Design review of the part shown in the three views and the two pictorial views. Dimensions are in mm from the part's minimum x, y and z. A direction names the side the tool comes from. Coordinates: 2 decimals unless noted, no trailing zeros. Loops run counter-clockwise (first coordinate to the right, second up) from the corner with the lowest first, then second, coordinate; pieces in that order, holes last.
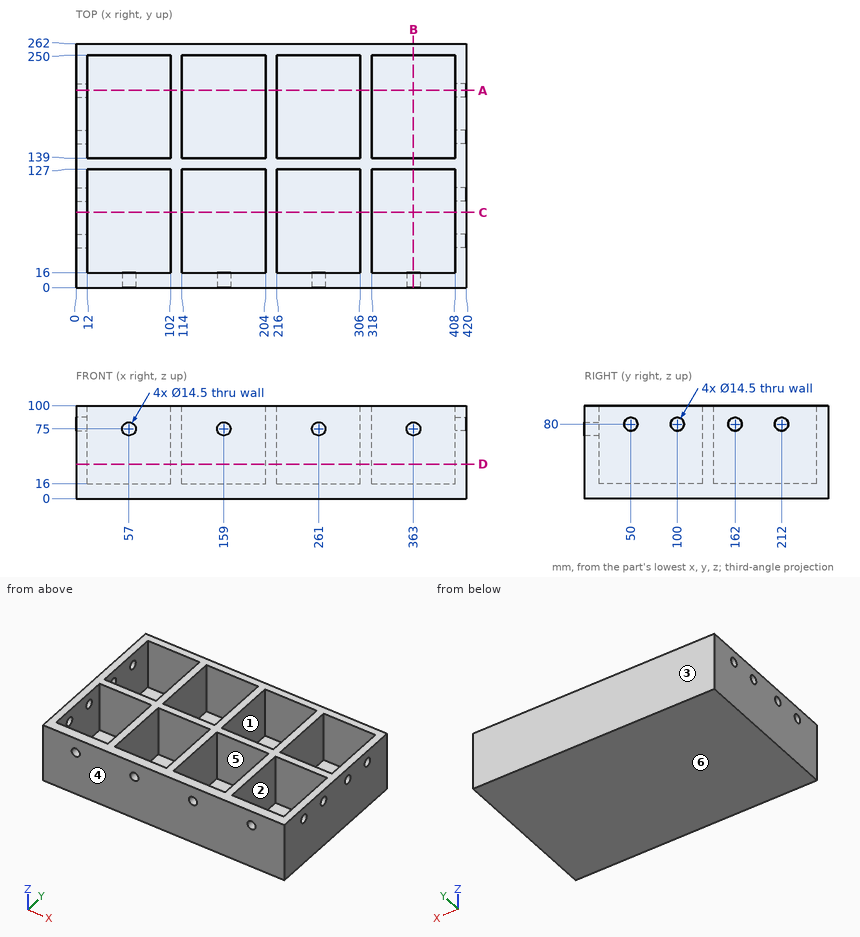
Q1. Wall thickness on probe 1 along X at (y, z) = (79.5, 85); probe 2 along X at (y, z) = (6, 75); probe 3 along Y at (x, z) = (164, 90): over which ranges is each line inside the solid? List them lowest first.
Q2. For pin 1 Ø8.5 at (x, z) = (57, 75) entering from -Y; pin 2 Ø1.5 at (x, y) = (79, 188) entering from +Z; pin 3 Ø11.5 at (y, z) = (162, 80) entering from +X, all flat-tipped, find the tip position at first contact; note any pin that passes through.
Q3. The part is to be moulded in two halves that separate along Y. For the marked faces 1, 2, 3 and 4, say which applies: +Y half, -Y half, draft (parallel to the pull), parting line (faces both ways), or undercut.
Q4. Consider section C-C (y = 81). State the section outline as (x, z) points, then the cut area to 3 significant figures.
Q5. Consider section B-B (x = 363). State the section outline as (y, z) points.
Q6. Consider section D-D (z = 37). Count the separate pieces of the cut face and the enclosed holes in it, then the cut area to 3 significant figures.
Q7. Consider section A-A (y = 212). State the section outline as (x, z) points, then the cut area to 3 significant figures.
Q8. Machinability: for the marked faces 5 and 6, which of the approach directions +Z, -Z, +X, -X, +Y, -Y give a long, thin tool a straight path to every point of the face, cutting with its end or side? Answer none if there is none.
Model answer:
1. probe 1: x = 0 to 12, 102 to 114, 204 to 216, 306 to 318, 408 to 420
1. probe 2: x = 0 to 49.75, 64.25 to 151.75, 166.25 to 253.75, 268.25 to 355.75, 370.25 to 420
1. probe 3: y = 0 to 16, 127 to 139, 250 to 262
2. pin 1: stops at y = 127
2. pin 2: stops at z = 16
2. pin 3: stops at x = 318
3. face 1: undercut
3. face 2: undercut
3. face 3: +Y half
3. face 4: -Y half
4. outline: (0, 0) - (420, 0) - (420, 100) - (408, 100) - (408, 16) - (318, 16) - (318, 100) - (306, 100) - (306, 16) - (216, 16) - (216, 100) - (204, 100) - (204, 16) - (114, 16) - (114, 100) - (102, 100) - (102, 16) - (12, 16) - (12, 100) - (0, 100) - close
4. area: 11,800 mm2
5. outline: (0, 0) - (262, 0) - (262, 100) - (250, 100) - (250, 16) - (139, 16) - (139, 100) - (127, 100) - (127, 16) - (16, 16) - (16, 67.75) - (0, 67.75) - close; (0, 82.25) - (16, 82.25) - (16, 100) - (0, 100) - close
6. separate pieces: 1
6. enclosed holes: 8
6. area: 30,100 mm2
7. outline: (0, 0) - (420, 0) - (420, 72.75) - (408, 72.75) - (408, 16) - (318, 16) - (318, 100) - (306, 100) - (306, 16) - (216, 16) - (216, 100) - (204, 100) - (204, 16) - (114, 16) - (114, 100) - (102, 100) - (102, 16) - (12, 16) - (12, 72.75) - (0, 72.75) - close; (0, 87.25) - (12, 87.25) - (12, 100) - (0, 100) - close; (408, 87.25) - (420, 87.25) - (420, 100) - (408, 100) - close
7. area: 11,400 mm2
8. face 5: +Z
8. face 6: -Z, +X, -X, +Y, -Y
